from build123d import *

# Parameters (mm, degrees)
F1_DEPTH = 6
F2_R     = 1.5
F3_DEPTH = 50.001
F4_R     = 2.99999
F5_SIZE  = 2.5


# Not quite as in the source:
# - a fillet or chamfer is up to 0.001 mm smaller than in the source, because OpenCascade refuses the exact size


with BuildPart() as f1:
    # F0 (on Top) → F1 (new body)
    with BuildSketch(Plane.XY):
        Polygon((0, 0), (0, -20), (50, -20), (50, 0), (40, 0), (40, -8), (10, -8), (10, 0), align=None)
    extrude(amount=F1_DEPTH)

    # F2 (on face) → F3 (cut, through all)
    with BuildSketch(Plane(origin=(0, 0, 0), x_dir=(0, -1, 0), z_dir=(-1, 0, 0))):
        with Locations((3.8, 3)):
            Circle(F2_R)
    extrude(amount=-F3_DEPTH, mode=Mode.SUBTRACT)

    # F4 (radius 3 in the source; OpenCascade refuses exactly that, so slightly less here)
    f4_edges = [f1.edges().sort_by_distance(p)[0] for p in [
        (5, 0, 6),
        (5, 0, 0),
        (45, 0, 6),
        (45, 0, 0),
        (25, -8, 6),
        (25, -8, 0),
    ]]
    fillet(f4_edges, radius=F4_R)

    # F5
    f5_edges = [f1.edges().sort_by_distance(p)[0] for p in [
        (25, -20, 0),
    ]]
    chamfer(f5_edges, length=F5_SIZE)


solid = f1.part
Could you check a few things on this model? Use its own coordinates, in mm. A direction names the side the tool comes from. Give positions to 0.01 mm unless a question says otherwise; leave off trailing zeros. Order: outer loops, then holes, each group sorted by start corner. A loop starts at its lowest first (then second) coordinate and runs counter-clockwise, first axis right, second up.
Item 1: If we section it at D-D, the plane z = 2: Write out the boundary of the cut face in (x, y).
Item 2: I need wall thicknesses on line 1 (Z direction, x = 46.25, y = -3.8); line 2 (Y direction, x = 3, z = 3.1); line 3 (X direction, y = -5.5, z = 4.7). Which ranges of each line are inside material? Lowest first, please.
Item 3: For faces 1 (the face through (24.79, -8.9, 5.14)), 2 (the face through (0, -10, 3)), 3 (the face through (24.79, -8.9, 0.86)), which set-ups out of +Z, -Z, +X, -X, +Y, -Y let a thin tool reach every point of the face, with its end or its side?
Item 4: If we section it at A-A, the plane y = -3.8: Write out the boundary of the cut face in (x, z).
Item 5: If we mould it in two halves opening along Z, with no side actions, what happens to faces 4 (the face through (44.9, -2.6, 2.1)), 5 (the face through (50, -10, 3)), 6 (the face through (4.93, -0.86, 0.9))? For each: pulls with the +Z half, pulls with the -Z half, needs draft (parallel to the pull), parting line crosses it, or undercut.
Item 6: I'm going to push a flat-ended pin straight in: pin 1 (2 mm diameter, centred on x = 20.5, z = 2, fed in from +Y). Where does the tip first touch, or does it pass through?
Item 7: If we section it at B-B, the plane y = -7: Write out the boundary of the cut face in (x, z), plus the area to 3 significant figures.
Values:
1. outline: (0, -19.5) - (50, -19.5) - (50, -4.92) - (40, -4.92) - (40, -8.17) - (10, -8.17) - (10, -4.92) - (0, -4.92) - close; (0, -2.68) - (10, -2.68) - (10, -0.17) - (0, -0.17) - close; (40, -2.68) - (50, -2.68) - (50, -0.17) - (40, -0.17) - close
2. line 1: z = 0 to 1.5, 4.5 to 6
2. line 2: y = -20 to -5.3, -2.3 to 0
2. line 3: x = 0 to 10, 40 to 50
3. face 1: +Z, +Y
3. face 2: +Z, -Z, -X, +Y, -Y
3. face 3: -Z, +Y
4. outline: (0, 0) - (10, 0) - (10, 1.5) - (0, 1.5) - close; (0, 4.5) - (10, 4.5) - (10, 6) - (0, 6) - close; (40, 0) - (50, 0) - (50, 1.5) - (40, 1.5) - close; (40, 4.5) - (50, 4.5) - (50, 6) - (40, 6) - close
5. face 4: undercut
5. face 5: needs draft
5. face 6: pulls with the -Z half
6. pin 1: stops at y = -8
7. outline: (0, 0) - (10, 0) - (10, 6) - (0, 6) - close; (40, 0) - (50, 0) - (50, 6) - (40, 6) - close
7. area: 120 mm2
